```python
from build123d import *

# Parameters (mm, degrees)
F0_R     = 11.2
F1_DEPTH = 7


# Not quite as in the source:
# - ends of sketch curves that miss each other by under 0.0002 mm in the source are joined


with BuildPart() as f1:
    # F0 (on Top) → F1 (new body)
    with BuildSketch(Plane.XY):
        with BuildLine():
            ThreePointArc((23.1851437088, -0.209827322), (11.4809905002, 6.6524743946), (11.4315817283, 20.219933477))
            ThreePointArc((11.4315817283, 20.219933477), (-9.27972e-05, 40.0198531118), (-11.4314889311, 20.2197727475))
            ThreePointArc((-11.4314889311, 20.2197727475), (-11.4807071504, 6.6523126094), (-23.1847645001, -0.2101533167))
            ThreePointArc((-23.1847645001, -0.2101533167), (-29.8083976459, -1.968183302), (-34.65797177, -6.8101680495))
            ThreePointArc((-34.65797177, -6.8101680495), (-29.8265597828, -24.8415250127), (-11.7950971191, -20.0105075285))
            ThreePointArc((-11.7950971191, -20.0105075285), (0.0002818311, -13.2693854266), (11.7957555615, -20.0103416826))
            ThreePointArc((11.7957555615, -20.0103416826), (29.8270373154, -24.8412493104), (34.6587334239, -6.8101809539))
            ThreePointArc((34.6587334239, -6.8101809539), (29.8271641279, -1.9786795899), (23.2271516953, -0.2102613183))
            ThreePointArc((23.2271516953, -0.2102613183), (23.2061475356, -0.2100604335), (23.1851437088, -0.209827322))
        make_face()
        with Locations((-23.2263900417, -13.4100876845)):
            Circle(F0_R, mode=Mode.SUBTRACT)
        Circle(F0_R, mode=Mode.SUBTRACT)
        with Locations((23.2269557018, -13.4097611005)):
            Circle(F0_R, mode=Mode.SUBTRACT)
        with Locations((0, 26.8198531121)):
            Circle(F0_R, mode=Mode.SUBTRACT)
        with BuildLine():
            ThreePointArc((34.6587334239, -6.8101809539), (29.8090523924, -1.9679079658), (23.1851437088, -0.209827322))
            ThreePointArc((23.1851437088, -0.209827322), (23.2061475356, -0.2100604335), (23.2271516953, -0.2102613183))
            ThreePointArc((23.2271516953, -0.2102613183), (29.8271641279, -1.9786795899), (34.6587334239, -6.8101809539))
        make_face()
        with BuildLine():
            ThreePointArc((11.7957555615, -20.0103416826), (29.8273248569, -24.8417502492), (34.6587334239, -6.8101809539))
            ThreePointArc((34.6587334239, -6.8101809539), (29.8270373154, -24.8412493104), (11.7957555615, -20.0103416826))
        make_face()
        with BuildLine():
            ThreePointArc((-11.7950971191, -20.0105075285), (-29.8265597828, -24.8415250127), (-34.65797177, -6.8101680495))
            ThreePointArc((-34.65797177, -6.8101680495), (-29.8268485884, -24.8420252217), (-11.7950971191, -20.0105075285))
        make_face()
    extrude(amount=F1_DEPTH)


solid = f1.part
```
Could you check a few things on this model? Use its own coordinates, in mm. Coordinates: 2 decimals unless noted, no trailing zeros. Loops run counter-clockwise (first coordinate to the right, second up) from the corner with the lowest first, then second, coordinate; pieces in that order, holes last. Notation, with made-up numbers: M -36.75,51 L -16.75,51 A19 ccw -16.75,60 Z; hole C 1.5,34.5 d2. An arc over 180 degrees is marked long. Put each result on its own line as item: value. Start each with the question number.
(1) Suppose I cut it at A-A on x = 0. Please give me the cut outline in (y, z), then the cut area to 3 significant figures.
(2) Will these pins go through, and if not, where does the flat tip stop? P1, Ø6, axis at x = 26.5, y = -5.5, coming from the +Z side; P2, Ø1.5, axis at x = -2, z = 3, coming from the +Y side; P3, Ø4, axis at y = -17, z = 1.5, coming from the +X side; P4, Ø1.5, axis at y = -2, z = 2.5, coming from the +X side.
(3) Thinking about a two-plate mould opening in X: for faces 1 (the face through (33.573, -17.699, 3.451)), 2 (the face through (-6, -10, 0)), 3 (the face through (11.58, 6.48, 3.45)), which applies, pulls with the +X half, pulls with the -X half, needs draft (parallel to the pull), parting line crosses it, or undercut?
(4) Suppose I cut it at C-C on x = 27.5. Please give me the cut outline in (y, z).
(5) Suppose I cut it at B-B on y = 28.5. Please give me the cut outline in (x, z).
(6) I need wall thicknesses on line 1 (X direction, y = -18, z = 5); line 2 (Y direction, x = 8, z = 1.75); line 3 (Y direction, x = 1, z = 1.25). Which ranges of each line are inside material? Lowest first, please. Write a range as from..to.
Solutions:
1. outline: M -13.27,0 L -11.2,0 L -11.2,7 L -13.27,7 Z; M 11.2,0 L 15.62,0 L 15.62,7 L 11.2,7 Z; M 38.02,0 L 40.02,0 L 40.02,7 L 38.02,7 Z
1. area: 59.4 mm2
2. P1: stops at z = 7
2. P2: stops at y = 39.96
2. P3: stops at x = 36.33
2. P4: stops at x = 31.01
3. face 1: undercut
3. face 2: needs draft
3. face 3: pulls with the +X half
4. outline: M -25.9,0 L -23.76,0 L -23.76,7 L -25.9,7 Z; M -3.06,0 L -0.92,0 L -0.92,7 L -3.06,7 Z
5. outline: M -13.09,0 L -11.07,0 L -11.07,7 L -13.09,7 Z; M 11.07,0 L 13.09,0 L 13.09,7 L 11.07,7 Z
6. line 1: x = -35.6..-33.44, -13.01..-10.35, 10.35..13.01, 33.44..35.6
6. line 2: y = -15.85..-7.84, 7.84..18.98, 34.66..37.32
6. line 3: y = -13.31..-11.16, 11.16..15.66, 37.98..39.98
